from build123d import *

# Parameters (mm, degrees)
SKETCH1_W               = 169
SKETCH1_H               = 7
BOSS_EXTRUDE1_DEPTH     = 109
SKETCH3_W               = 165
SKETCH3_H               = 105
CUT_EXTRUDE2_DEPTH      = 1.5
SKETCH4_W               = 84.5
SKETCH4_H               = 1.55
CUT_EXTRUDE3_DEPTH      = 2
SKETCH5_R               = 2.5
BOSS_EXTRUDE2_DEPTH     = 8
SKETCH6_R               = 2.5
BOSS_EXTRUDE3_DEPTH     = 8
SKETCH8_W               = 10
SKETCH8_H               = 15
BOSS_EXTRUDE4_DEPTH     = 10
SKETCH9_R               = 2.55
CUT_EXTRUDE4_DEPTH      = 35.1
CUT_EXTRUDE4_DEPTH_BACK = 5.1
SKETCH10_W              = 167
SKETCH10_H              = 107
CUT_EXTRUDE5_DEPTH      = 1.55


with BuildPart() as part:
    # Sketch1 → Boss-Extrude1 (new body)
    with BuildSketch(Plane.XY):
        with Locations((84.5, 3.5)):
            Rectangle(SKETCH1_W, SKETCH1_H)
    extrude(amount=-BOSS_EXTRUDE1_DEPTH)

    # Sketch3 → Cut-Extrude2 (cut)
    with BuildSketch(Plane(origin=(0, 7, 0), x_dir=(1, 0, 0), z_dir=(0, 1, 0))):
        with Locations((84.5, 54.5)):
            Rectangle(SKETCH3_W, SKETCH3_H)
    extrude(amount=-CUT_EXTRUDE2_DEPTH, mode=Mode.SUBTRACT)

    # Sketch4 → Cut-Extrude3 (cut)
    with BuildSketch(Plane.XY):
        with Locations((84.5, 6.225)):
            Rectangle(SKETCH4_W, SKETCH4_H)
    extrude(amount=-CUT_EXTRUDE3_DEPTH, mode=Mode.SUBTRACT)

    # Sketch5 → Boss-Extrude2 (add)
    with BuildSketch(Plane(origin=(169, 0, 0), x_dir=(0, 0, -1), z_dir=(1, 0, 0))):
        with Locations((54.5, 3.5)):
            Circle(SKETCH5_R)
    extrude(amount=BOSS_EXTRUDE2_DEPTH)

    # Sketch6 → Boss-Extrude3 (add)
    with BuildSketch(Plane(origin=(0, 0, -109), x_dir=(-1, 0, 0), z_dir=(0, 0, -1))):
        with Locations((-84.5, 3.5)):
            Circle(SKETCH6_R)
    extrude(amount=BOSS_EXTRUDE3_DEPTH)

    # Sketch8 → Boss-Extrude4 (add)
    with BuildSketch(Plane.XZ):
        with Locations((104.5, -54.5)):
            Rectangle(SKETCH8_W, SKETCH8_H)
        with Locations((64.5, -54.5)):
            Rectangle(SKETCH8_W, SKETCH8_H)
    extrude(amount=BOSS_EXTRUDE4_DEPTH)

    # Sketch9 → Cut-Extrude4 (cut, two sides)
    with BuildSketch(Plane(origin=(69.5, 0, 0), x_dir=(0, 0, -1), z_dir=(1, 0, 0))) as cut_extrude4_sk:
        with Locations((54.5, -10)):
            Circle(SKETCH9_R)
    extrude(amount=CUT_EXTRUDE4_DEPTH, mode=Mode.SUBTRACT)
    extrude(cut_extrude4_sk.sketch, amount=-CUT_EXTRUDE4_DEPTH_BACK, mode=Mode.SUBTRACT)

    # Sketch10 → Cut-Extrude5 (cut)
    with BuildSketch(Plane(origin=(0, 7, 0), x_dir=(1, 0, 0), z_dir=(0, 1, 0))):
        with Locations((84.5, 54.5)):
            Rectangle(SKETCH10_W, SKETCH10_H)
    extrude(amount=-CUT_EXTRUDE5_DEPTH, mode=Mode.SUBTRACT)


solid = part.part
Design review of the part built by this model. Coordinates are the model's own, in mm. A direction names the side the tool comes from. Round coordinates to 2 decimals unless told otherwise and drop trailing zeros. Write each loop counter-clockwise with the first axis right and the second up, starting at its lowest first coordinate (ties: lowest second). Pieces come first, ordered by that corner, then holes. Notation, with made-up numbers: M 51.25,-38 L 77.25,-38 A14 ccw 77.25,-28 Z; hole C 4.25,87.25 d11. An arc over 180 degrees is marked long. One line per item, written item: value. Start each with the question number.
1. Draft analysis for pull direction X (two halves, no side actions). For faces 1 (the face through (0, 3, -54)), 2 (the face through (83, 5.45, -53)), 3 (the face through (172.94, 2.54, -56.81)), 4 (the face through (177, 4, -54)), state which applies: pulls with the +X half, pulls with the -X half, needs draft (parallel to the pull), parting line crosses it, or undercut.
2. Take a section at D-D on x = 84.5. State the section outline as (y, z) points, then the cut area to 3 significant figures.
3. Take a section at C-C on z = -54.5. State the section outline as (x, y) points, then the cut area to 3 significant figures.
4. For faces 5 (the face through (109.5, -5, -55)), 6 (the face through (59.5, -5, -55)), 7 (the face through (64, -5, -47)), 8 (the face through (64, -5, -62)), 9 (the face through (87, 3.6, -112.9)), list the 3-axis set-ups (+Z, -Z, +X, -X, +Y, -Y) from which the entire face can be reached by the end or side of a thin tool; tool diameter is ignored.
5. Take a section at B-B on x = 157.5. State the section outline as (y, z) points, then the cut area to 3 significant figures.
6. To check wall thickness, follow probe 1 along Y at (x, z) = (17, -93); probe 2 along X at (y, z) = (4.75, -45); probe 3 along Z at (x, y) = (64, -3). State the ranges of each line that lie inside material, in increasing order. Write a range as from..to.
7. Clearance check with flat-ended pins moving along their axes: P1, Ø1.7, axis at x = 30, y = 6, coming from the -Z side; P2, Ø7.5, axis at y = 5, z = -44.5, coming from the +X side; P3, Ø3, axis at y = -3.5, z = -52.5, coming from the -X side. State where each tip first meets the part, or that it passes through.
8. Take a section at A-A on y = -3. State the section outline as (x, z) points, then the cut area to 3 significant figures.
Computed:
1. face 1: pulls with the -X half
1. face 2: undercut
1. face 3: needs draft
1. face 4: pulls with the +X half
2. outline: M 0,-109 L 1,-109 L 1,-117 L 6,-117 L 6,-109 L 7,-109 L 7,-108 L 5.45,-108 L 5.45,0 L 0,0 Z
2. area: 636 mm²
3. outline: M 0,0 L 59.5,0 L 59.5,-10 L 64.4,-10 L 64.4,-7.45 L 69.5,-7.45 L 69.5,0 L 99.5,0 L 99.5,-7.45 L 104.6,-7.45 L 104.6,-10 L 109.5,-10 L 109.5,0 L 169,0 L 169,1 L 177,1 L 177,6 L 169,6 L 169,7 L 168,7 L 168,5.45 L 1,5.45 L 1,7 L 0,7 Z
3. area: 1,140 mm²
4. face 5: +Z, -Z, +X, -Y
4. face 6: +Z, -Z, -X, -Y
4. face 7: +Z, +X, -X, -Y
4. face 8: -Z, +X, -X, -Y
4. face 9: -Z
5. outline: M 0,-109 L 7,-109 L 7,-108 L 5.45,-108 L 5.45,-1 L 7,-1 L 7,0 L 0,0 Z
5. area: 597 mm²
6. probe 1: y = 0..5.45
6. probe 2: x = 0..169
6. probe 3: z = -62..-47
7. P1: stops at z = -109
7. P2: stops at x = 169
7. P3: stops at x = 59.5
8. outline: M 59.5,-62 L 69.5,-62 L 69.5,-47 L 59.5,-47 Z; M 99.5,-62 L 109.5,-62 L 109.5,-47 L 99.5,-47 Z
8. area: 300 mm²
